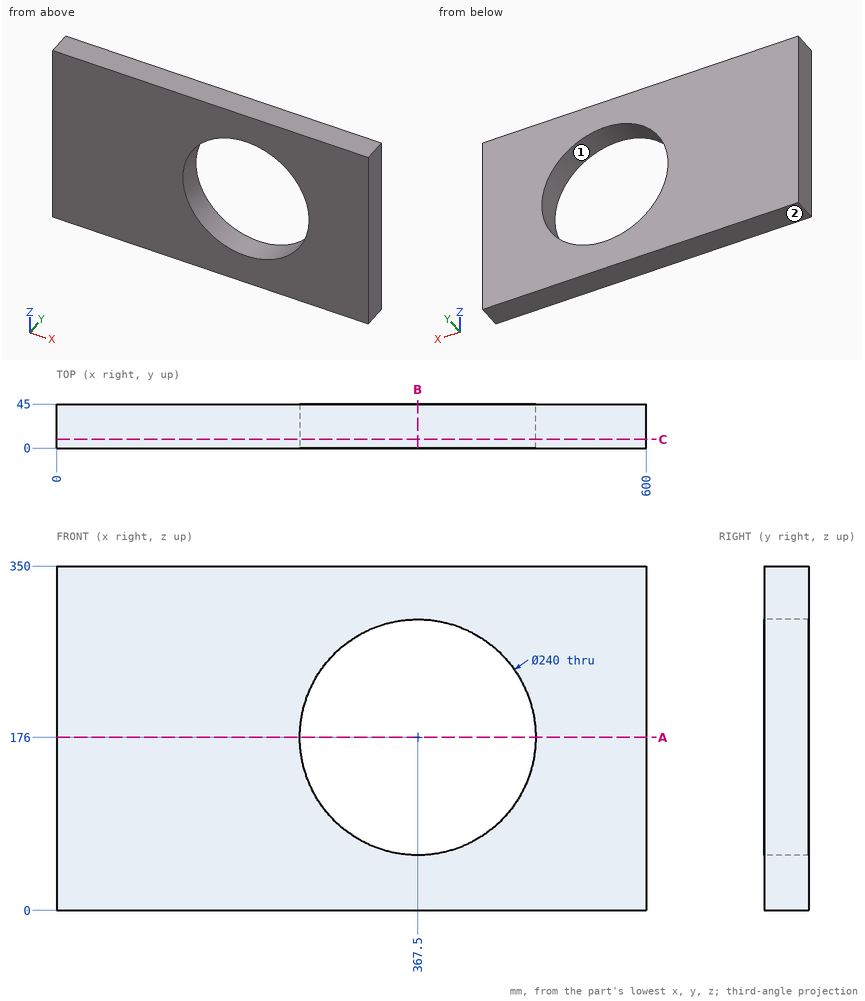
Drawing for the job (mm, zero at the part's lowest x, y, z). Round coordinates to 2 decimals unless told otherwise and drop trailing zeros. Loops run counter-clockwise (first coordinate to the right, second up) from the corner with the lowest first, then second, coordinate; pieces in that order, holes last. Notation, with made-up numbers: (-37, 44.5) - (-24, 44.5) arc R18 cw to (-24, 67.5) - close; hole circle Ø5 at (38, 17). An arc over 180 degrees is marked (long way). Return JSON: item names as keys, results as strings. Group by question number.
Q1. Drill centre lines: line 1 along X through (y, z) = (33.5, 176); line 2 along Z through (x, y) = (367.5, 10); line 3 along X through (y, z) = (8, 85). Where is each one in solid material? Low to high. Write a range as [from, to].
Q2. Band-saw the part on B-B on x = 367.5. Give the cut face in (y, z), plus the area to 3 significant figures.
Q3. Band-saw the part on A-A on z = 176. Give the cut face in (x, y), plus the area to 3 significant figures.
Q4. Band-saw the part on C-C on y = 9. Give the cut face in (x, z).
Q5. Two-plate mould, pull along X, no slides. Class the marked faces 1 and 2: +X half, -X half, draft (parallel to the pull), parting line (faces both ways), or undercut.
Solutions:
{
 "1": {"line 1": "x = [0, 247.5], [487.5, 600]", "line 2": "z = [0, 56], [296, 350]", "line 3": "x = [0, 289.28], [445.72, 600]"},
 "2": {"outline": "(0, 0) - (45, 0) - (45, 56) - (0, 56) - close; (0, 296) - (45, 296) - (45, 350) - (0, 350) - close", "area": "4,950 mm^2"},
 "3": {"outline": "(0, 0) - (247.5, 0) - (247.5, 45) - (0, 45) - close; (487.5, 0) - (600, 0) - (600, 45) - (487.5, 45) - close", "area": "16,200 mm^2"},
 "4": {"outline": "(0, 0) - (600, 0) - (600, 350) - (0, 350) - close; hole circle Ø240 at (367.5, 176)"},
 "5": {"face 1": "undercut", "face 2": "draft"}
}
